from build123d import *

# Parameters (mm, degrees)
SKETCH1_W           = 150
SKETCH1_H           = 130
BOSS_EXTRUDE1_DEPTH = 3
SKETCH2_R           = 1.6
CUT_EXTRUDE1_DEPTH  = 23
SKETCH3_W           = 50
SKETCH3_H           = 15
SKETCH3_H_2         = 16
BOSS_EXTRUDE2_DEPTH = 3


with BuildPart() as part:
    # Sketch1 → Boss-Extrude1 (new body)
    with BuildSketch(Plane.XY):
        Rectangle(SKETCH1_W, SKETCH1_H)
    extrude(amount=BOSS_EXTRUDE1_DEPTH)

    # Sketch2 → Cut-Extrude1 (cut)
    with BuildSketch(Plane.XY.offset(3)):
        with Locations((63, 57)):
            Circle(SKETCH2_R)
        with Locations((70.5, 5)):
            Circle(SKETCH2_R)
        with Locations((-5, 57)):
            Circle(SKETCH2_R)
        with Locations((-5, -32)):
            Circle(SKETCH2_R)
        with Locations((63, -32)):
            Circle(SKETCH2_R)
        with Locations((70.5, -5)):
            Circle(SKETCH2_R)
        with Locations((-18, 57)):
            Circle(SKETCH2_R)
        with Locations((-18, 8.4)):
            Circle(SKETCH2_R)
        with Locations((-55.3, 8.4)):
            Circle(SKETCH2_R)
        with Locations((-55.3, 57)):
            Circle(SKETCH2_R)
        with Locations((-18, -57)):
            Circle(SKETCH2_R)
        with Locations((-55.3, -57)):
            Circle(SKETCH2_R)
        with Locations((-55.3, -8.4)):
            Circle(SKETCH2_R)
        with Locations((-18, -8.4)):
            Circle(SKETCH2_R)
        with Locations((-30.4, 58.5)):
            Circle(SKETCH2_R)
        with Locations((-68.4, 58.5)):
            Circle(SKETCH2_R)
        with Locations((-68.4, 48.5)):
            Circle(SKETCH2_R)
        with Locations((-30.4, 48.5)):
            Circle(SKETCH2_R)
        with Locations((-68.4, -48.5)):
            Circle(SKETCH2_R)
        with Locations((-68.4, -58.5)):
            Circle(SKETCH2_R)
        with Locations((-30.4, -58.5)):
            Circle(SKETCH2_R)
        with Locations((-30.4, -48.5)):
            Circle(SKETCH2_R)
        with Locations((-69, -30)):
            Circle(SKETCH2_R)
        with Locations((-69, 30)):
            Circle(SKETCH2_R)
        with Locations((-55.3, 37)):
            Circle(SKETCH2_R)
        with Locations((-55.3, -37)):
            Circle(SKETCH2_R)
    extrude(amount=-CUT_EXTRUDE1_DEPTH, mode=Mode.SUBTRACT)

    # Sketch3 → Boss-Extrude2 (add)
    with BuildSketch(Plane(origin=(0, 0, 0), x_dir=(-1, 0, 0), z_dir=(0, 0, -1))):
        with Locations((50, 72.5)):
            Rectangle(SKETCH3_W, SKETCH3_H)
        with Locations((50, -73)):
            Rectangle(SKETCH3_W, SKETCH3_H_2)
    extrude(amount=-BOSS_EXTRUDE2_DEPTH)


solid = part.part
The listing builds one solid part. Answer for the finished solid, in the listing's coordinates (mm). Round coordinates to 2 decimals unless told otherwise and drop trailing zeros. Loops run counter-clockwise (first coordinate to the right, second up) from the corner with the lowest first, then second, coordinate; pieces in that order, holes last. Notation, with made-up numbers: M 55,-11.75 L 63,-11.75 A23 cw 63,16.25 Z; hole C 37,11.25 d10. An arc over 180 degrees is marked long. Write each question's results on one line, items separated by ' | '. Start each with the question number.
1) Find section C-C on x = 20. Write down the section's boundary in (y, z).
2) Find section A-A on z = 1.4. Count the separate pieces of the cut face and the enclosed holes in it, plus the area to 3 significant figures.
3) Straight lines are drawn through the part: probe 1 along Y at (x, z) = (-18, 0.6); probe 2 along Y at (x, z) = (63, 0.9); probe 3 along X at (y, z) = (-67.5, 2.25). For each, find the intervals that lie inside material, in ascending order.
4) Find section B-B on y = 67.5. Write down the section's boundary in (x, z), plus the area to 3 significant figures.
5) Each of these flat-tipped pins is pushed along its axis until it touches: pin 1 (0.9 mm diameter, centred on y = -76, z = 2, fed in from +X); pin 2 (4 mm diameter, centred on x = -13.5, y = -37, fed in from -Z); pin 3 (1.9 mm diameter, centred on x = -55.3, y = 37, fed in from +Z). Where does it stop, or does it pass through?
Final values:
1) outline: M -65,0 L 65,0 L 65,3 L -65,3 Z
2) separate pieces: 1 | enclosed holes: 26 | area: 20,800 mm²
3) probe 1: -65 to -58.6, -55.4 to -10, -6.8 to 6.8, 10 to 55.4, 58.6 to 65 | probe 2: -65 to -33.6, -30.4 to 55.4, 58.6 to 65 | probe 3: -75 to -25
4) outline: M -75,0 L -25,0 L -25,3 L -75,3 Z | area: 150 mm²
5) pin 1: x = -25 | pin 2: z = 0 | pin 3: through
